Part model, mm, in its own coordinate system. Coordinates: 2 decimals unless noted, no trailing zeros. Write each loop counter-clockwise with the first axis right and the second up, starting at its lowest first coordinate (ties: lowest second). Pieces come first, ordered by that corner, then holes. Notation, with made-up numbers: (-35.75, 80) -> (-20.75, 80) arc R19 ccw to (-20.75, 88) -> close; hole circle Ø5 at (54, -22.5). An arc over 180 degrees is marked (long way). One line per question, with ' | ' between items. Start each with the question number.
Item 1: Saw through at C-C (x = 0). List the corners of the cut face in (y, z), and give its area (3 significant figures).
Item 2: Saw through at D-D (z = 0.75). List the corners of the cut face in (x, y), and give its area (3 significant figures).
Item 3: Probe probe 1 along Y at (x, z) = (0, 1.1); probe 2 along Y at (x, z) = (-15.5, 1.75); probe 3 along X at (y, z) = (19, 1.35). List the from-to ranges inside material, lowest first. Write a range as [from, to].
Item 4: Saw through at B-B (y = 0). List the corners of the cut face in (x, z), and give its area (3 significant figures).
Item 5: Saw through at A-A (x = 15.6). List the corners of the cut face in (y, z).
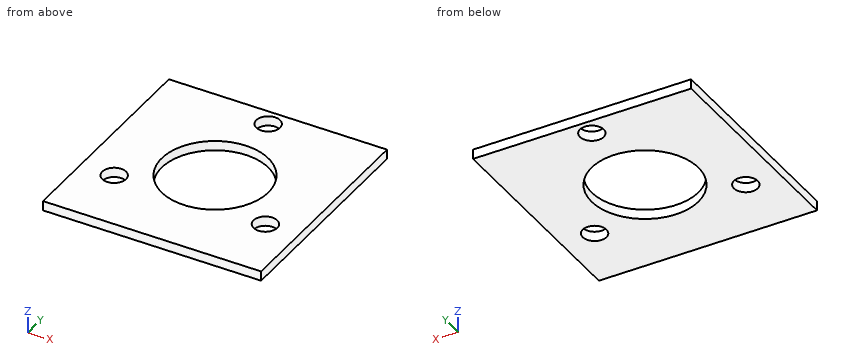
Autodesk Inventor part; units mm, degrees
ref_plane "YZ Plane" through (0, 0, 0) normal (1, 0, 0) x (0, 1, 0)
ref_plane "XZ Plane" through (0, 0, 0) normal (0, 1, 0) x (-1, 0, 0)
ref_plane "XY Plane" through (0, 0, 0) normal (0, 0, 1) x (1, 0, 0)
sketch "Sketch1" plane through (0, 0, 0) normal (0, 0, 1) x (1, 0, 0)
  line L0 (-22.5, -22.5) -> (22.5, -22.5)
  line L1 (22.5, -22.5) -> (22.5, 22.5)
  line L2 (22.5, 22.5) -> (-22.5, 22.5)
  line L3 (-22.5, 22.5) -> (-22.5, -22.5)
  line L4 (-22.5, -22.5) -> (22.5, 22.5) construction
  line L5 (22.5, -22.5) -> (-22.5, 22.5) construction
  circle A0 centre (0, 0) radius 11
  line L6 (0, 0) -> (0, 19)
  line L7 (0, 0) -> (15.6, -9.0067)
  line L8 (0, 0) -> (-15.6, -9.0067)
  circle A1 centre (0, 19) radius 2.45
  circle A2 centre (15.6, -9.0067) radius 2.45
  circle A3 centre (-15.6, -9.0067) radius 2.45
  point P0 (22.5, -11.0947)
  point P1 (-22.5, -11.0947)
  dimension "d0" = 45
  dimension "d1" = 45
  dimension "d2" = 22
  dimension "d3" = 19
  dimension "d4" = 15.6
  dimension "d5" = 120
  dimension "d6" = 15.6
  dimension "d7" = 120
  dimension "d8" = 4.9
  dimension "d9" = 4.9
  dimension "d10" = 4.9
extrude "Extrusion2" add sketch "Sketch1" along normal blind 2
equation "\"d1\" = d0"
equation "\"d4\" = d6"
equation "\"d7\" = d5"
equation "\"d9\" = d8"
equation "\"d10\" = d8"
properties part number "mount_v06"
From the geometry:
1) outline: (-22.5, 0) -> (-11, 0) -> (-11, 2) -> (-22.5, 2) -> close; (11, 0) -> (16.55, 0) -> (16.55, 2) -> (11, 2) -> close; (21.45, 0) -> (22.5, 0) -> (22.5, 2) -> (21.45, 2) -> close | area: 36.2 mm2
2) outline: (-22.5, -22.5) -> (22.5, -22.5) -> (22.5, 22.5) -> (-22.5, 22.5) -> close; hole circle Ø4.9 at (-15.6, -9.01); hole circle Ø22 at (0, 0); hole circle Ø4.9 at (0, 19); hole circle Ø4.9 at (15.6, -9.01) | area: 1,590 mm2
3) probe 1: [-22.5, -11], [11, 16.55], [21.45, 22.5] | probe 2: [-22.5, -11.45], [-6.56, 22.5] | probe 3: [-22.5, -2.45], [2.45, 22.5]
4) outline: (-22.5, 0) -> (-11, 0) -> (-11, 2) -> (-22.5, 2) -> close; (11, 0) -> (22.5, 0) -> (22.5, 2) -> (11, 2) -> close | area: 46.0 mm2
5) outline: (-22.5, 0) -> (-11.46, 0) -> (-11.46, 2) -> (-22.5, 2) -> close; (-6.56, 0) -> (22.5, 0) -> (22.5, 2) -> (-6.56, 2) -> close
